from build123d import *

# Parameters (mm, degrees)
SKETCH5_W            = 75
SKETCH5_H            = 40
SKETCH5_R            = 2.5
BOSS_EXTRUDE6_DEPTH  = 10
SKETCH6_W            = 125
SKETCH6_H            = 40
BOSS_EXTRUDE7_DEPTH  = 10
SKETCH7_W            = 125
SKETCH7_H            = 40
BOSS_EXTRUDE8_DEPTH  = 10
SKETCH8_R            = 2.5
BOSS_EXTRUDE9_DEPTH  = 11.55
SKETCH10_R           = 3
SKETCH10_R_2         = 2.5
BOSS_EXTRUDE10_DEPTH = 11.55


with BuildPart() as part:
    # Sketch5 → Boss-Extrude6 (new body)
    with BuildSketch(Plane(origin=(0, 0, 0), x_dir=(0, 0, -1), z_dir=(1, 0, 0))):
        Rectangle(SKETCH5_W, SKETCH5_H)
        Circle(SKETCH5_R, mode=Mode.SUBTRACT)
    extrude(amount=BOSS_EXTRUDE6_DEPTH)

    # Sketch6 → Boss-Extrude7 (add)
    with BuildSketch(Plane(origin=(0, 0, -37.5), x_dir=(-1, 0, 0), z_dir=(0, 0, -1))):
        with Locations((-62.5, 0)):
            Rectangle(SKETCH6_W, SKETCH6_H)
    extrude(amount=-BOSS_EXTRUDE7_DEPTH)

    # Sketch7 → Boss-Extrude8 (add)
    with BuildSketch(Plane.XY.offset(37.5)):
        with Locations((62.5, 0)):
            Rectangle(SKETCH7_W, SKETCH7_H)
    extrude(amount=-BOSS_EXTRUDE8_DEPTH)

    # Sketch8 → Boss-Extrude9 (add)
    with BuildSketch(Plane(origin=(0, 0, -37.5), x_dir=(-1, 0, 0), z_dir=(0, 0, -1))):
        with Locations((-62.5, 0)):
            Circle(SKETCH8_R)
    extrude(amount=BOSS_EXTRUDE9_DEPTH)

    # Sketch10 → Boss-Extrude10 (add)
    with BuildSketch(Plane(origin=(0, 0, 37.5), x_dir=(-1, 0, 0), z_dir=(0, 0, -1))):
        with Locations((-62.5, 0)):
            Circle(SKETCH10_R)
        with Locations((-62.5, 0)):
            Circle(SKETCH10_R_2, mode=Mode.SUBTRACT)
    extrude(amount=-BOSS_EXTRUDE10_DEPTH)


solid = part.part
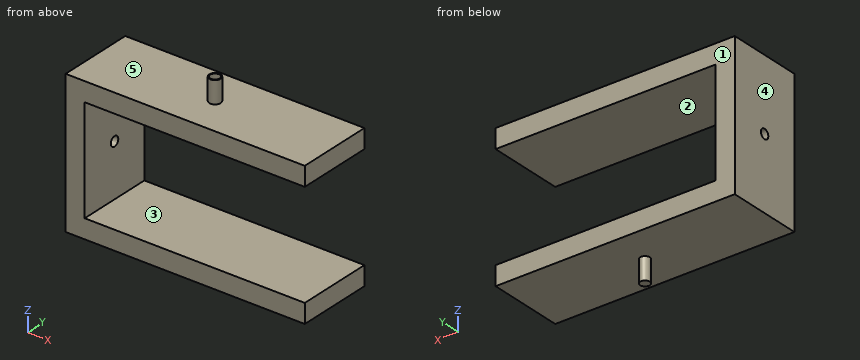
Input: part model. Units: mm. Frame: model coordinates. Face numbers are marked on the shaded views. A direction names the side the tool comes from. Round coordinates to 2 decimals unless told otherwise and drop trailing zeros. Loops run counter-clockwise (first coordinate to the right, second up) from the corner with the lowest first, then second, coordinate; pieces in that order, holes last. Notation, with made-up numbers: (19, 53) -> (38, 53) arc R33 ccw to (38, 83) -> close; hole circle Ø9 at (89, -4). An arc over 180 degrees is marked (long way). Answer as a JSON object with one key per item and string values. Group by question number.
1) Section query A-A on z = 0. Output: boundary loops of the cut face in (x, y).
2) Pin query (flat end, axial travel): pin 1 (4 mm diameter, centred on y = -0.5, z = -0.5, fed in from +X); pin 2 (1.5 mm diameter, centred on x = 61.5, y = 0, fed in from +Z); pin 3 (12 mm diameter, centred on x = 95.5, y = -2.5, fed in from -Z); pin 4 (4 mm diameter, centred on y = 0, z = 0, fed in from +X). Return the tip coordinate at first contact, or that it passes through.
3) Reachability of the marked faces 1 and 2 from +Z, -Z, +X, -X, +Y, -Y: full face, straight path, thin tool, end or side. Return the list, or none.
4) Draft query along Z for the marked faces 3, 4 and 5. Return one class per face: +Z half, -Z half, draft (parallel to the pull), parting line (faces both ways), or undercut.
5) Section query B-B on x = 94. Output: boundary loops of the cut face in (y, z), plus the area to 3 significant figures.
6) Section query C-C on y = 0. Output: boundary loops of the cut face in (x, z), plus the area to 3 significant figures.
7) Section query D-D on y = -7.5. Output: boundary loops of the cut face in (x, z).
8) Ray query, L1, parallel to Y at x = 7.25, z = 0; L2, parallel to Z at x = 13.5, y = 13; L3, parallel to Y at x = 62.5, z = 43.25. Return the intervals inside material, ascending.
Reply:
{
 "1": {"outline": "(0, -20) -> (10, -20) -> (10, -2.5) -> (0, -2.5) -> close; (0, 2.5) -> (10, 2.5) -> (10, 20) -> (0, 20) -> close"},
 "2": {"pin 1": "stops at x = 10", "pin 2": "stops at z = 37.5", "pin 3": "stops at z = -37.5", "pin 4": "passes through"},
 "3": {"face 1": "+Z, -Z, +X, -X, +Y", "face 2": "+X, +Y, -Y"},
 "4": {"face 3": "undercut", "face 4": "draft", "face 5": "+Z half"},
 "5": {"outline": "(-20, -37.5) -> (20, -37.5) -> (20, -27.5) -> (-20, -27.5) -> close; (-20, 27.5) -> (20, 27.5) -> (20, 37.5) -> (-20, 37.5) -> close", "area": "800 mm2"},
 "6": {"outline": "(0, -37.5) -> (60, -37.5) -> (60, -49.05) -> (65, -49.05) -> (65, -37.5) -> (125, -37.5) -> (125, -27.5) -> (10, -27.5) -> (10, -2.5) -> (0, -2.5) -> close; (0, 2.5) -> (10, 2.5) -> (10, 27.5) -> (125, 27.5) -> (125, 37.5) -> (65.5, 37.5) -> (65.5, 49.05) -> (65, 49.05) -> (65, 37.5) -> (60, 37.5) -> (60, 49.05) -> (59.5, 49.05) -> (59.5, 37.5) -> (0, 37.5) -> close", "area": "3,070 mm2"},
 "7": {"outline": "(0, -37.5) -> (125, -37.5) -> (125, -27.5) -> (10, -27.5) -> (10, 27.5) -> (125, 27.5) -> (125, 37.5) -> (0, 37.5) -> close"},
 "8": {"L1": "y = -20 to -2.5, 2.5 to 20", "L2": "z = -37.5 to -27.5, 27.5 to 37.5", "L3": "y = -3 to -2.5, 2.5 to 3"}
}
